Build history of the part. All positions in model axes, mm. A direction names the side the tool comes from. Give positions to 0.01 mm unless a question says otherwise; leave off trailing zeros. Write each loop counter-clockwise with the first axis right and the second up, starting at its lowest first coordinate (ties: lowest second). Pieces come first, ordered by that corner, then holes. Notation, with made-up numbers: (70, 41.25) -> (75, 41.25) arc R11 cw to (75, 60.25) -> close; hole circle Ø9 at (21, 41). An arc over 180 degrees is marked (long way). One line per question, with ' | ' between items. Start each with the question number.
(1) Band-saw the part on A-A, the plane y = -19.75. Give the cut face in (x, z) (3 decimals).
(2) Pin check, flat tips, straight feed: P1, Ø12.5, axis at x = 25, y = -8, coming from the -Z side (3 decimals); P2, Ø2, axis at y = -9.5, z = -1, coming from the +X side; P3, Ø7.5, axis at x = 25.5, y = -11, coming from the +Z side. Stop position of each tip, or through.
(3) Band-saw the part on C-C, the plane x = 30. Give the cut face in (y, z) (3 decimals).
(4) Pull direction X, two halves, no side cores. Call faces 1 (the cylindrical face through (-35.75, -12.52, 56.46)), 2 (the flat face through (38.1, -13, 54)), 3 (the flat face through (-40, -25.4, 12)): released by +X, released by -X, zero draft, split by the parting line, or undercut.
(5) Drill centre lines: probe 1 along Z at (x, y) = (28, -9.75) (3 decimals); probe 2 along X at (y, z) = (-17.75, 71); probe 3 along X at (y, z) = (-11.25, 53.5). Where is each one in solid material? Low to high. Write a range as from..to.
(6) Band-saw the part on B-B, the plane z = -15.5. Give the cut face in (x, y), and give its area (3 significant figures).
(7) Tool access for faces 4 (the flat face through (-53, -13, -30.327)), 5 (the flat face through (51, -13, 51.937)), 6 (the flat face through (26, -13, 67.1)), 7 (the cylindrical face through (4.356, -12.522, 47.991)), 8 (the flat face through (-104.173, -13, -15)): list every direction of +Z, -Z, +X, -X, +Y, -Y with a clear straight run to the whole face (end or side of a thin tool).
from build123d import *

# Parameters (mm, degrees)
F1_DEPTH = 25.4


with BuildPart() as f1:
    # F0 (on Front) → F1 (new body)
    with BuildSketch(Plane.XZ):
        Polygon((0, -30.327365), (0, 0), (-76.2, 0), (-104.173273, 0), (-104.173273, -30.327365), align=None)
        Polygon((-76.2, 0), (0, 0), (0, 25.4), (-11.711787, 25.4), (-76.2, 25.4), align=None)
        with BuildLine():
            Line((-104.173273, 0), (-76.2, 0))
            Line((-76.2, 0), (-76.2, 25.4))
            ThreePointArc((-76.2, 25.4), (-87.233659, 9.447856), (-104.173273, 0))
        make_face()
        with BuildLine():
            Line((-11.711787, 25.4), (0, 25.4))
            Line((0, 25.4), (0, 38.1))
            ThreePointArc((0, 38.1), (4.447352, 48.115325), (12.7, 55.325005))
            Line((12.7, 55.325005), (38.1, 55.325005))
            Line((38.1, 55.325005), (38.1, 67.100359))
            Line((38.1, 67.100359), (12.7, 67.100359))
            ThreePointArc((12.7, 67.100359), (-3.36853, 55.851652), (-11.711787, 38.1))
            Line((-11.711787, 38.1), (-11.711787, 25.4))
        make_face()
        with BuildLine():
            ThreePointArc((12.7, 67.100359), (-36.397174, 56.157378), (-76.2, 25.4))
            Line((-76.2, 25.4), (-11.711787, 25.4))
            Line((-11.711787, 25.4), (-11.711787, 38.1))
            ThreePointArc((-11.711787, 38.1), (-3.36853, 55.851652), (12.7, 67.100359))
        make_face()
        Polygon((38.1, 77.336693), (38.1, 67.100359), (38.1, 55.325005), (38.1, 51.936693), (63.5, 51.936693), (63.5, 77.336693), align=None)
    extrude(amount=F1_DEPTH)


solid = f1.part
Results:
1) outline: (-104.173, -30.327) -> (0, -30.327) -> (0, 38.1) arc R25.4 cw to (12.7, 55.325) -> (38.1, 55.325) -> (38.1, 51.937) -> (63.5, 51.937) -> (63.5, 77.337) -> (38.1, 77.337) -> (38.1, 67.1) -> (12.7, 67.1) arc R115.612 ccw to (-76.2, 25.4) arc R42.822 cw to (-104.173, 0) -> close
2) P1: stops at z = 55.325 | P2: stops at x = 0 | P3: stops at z = 67.1
3) outline: (-25.4, 55.325) -> (0, 55.325) -> (0, 67.1) -> (-25.4, 67.1) -> close
4) face 1: released by -X | face 2: undercut | face 3: zero draft
5) probe 1: z = 55.325..67.1 | probe 2: x = 38.1..63.5 | probe 3: x = -41.7..9.84, 38.1..63.5
6) outline: (-104.17, -25.4) -> (0, -25.4) -> (0, 0) -> (-104.17, 0) -> close | area: 2,650 mm²
7) face 4: -Z, +X, -X, +Y, -Y | face 5: -Z, +X, +Y, -Y | face 6: +Z, -X, +Y, -Y | face 7: -Z, +Y, -Y | face 8: +Z, -Z, -X, +Y, -Y
